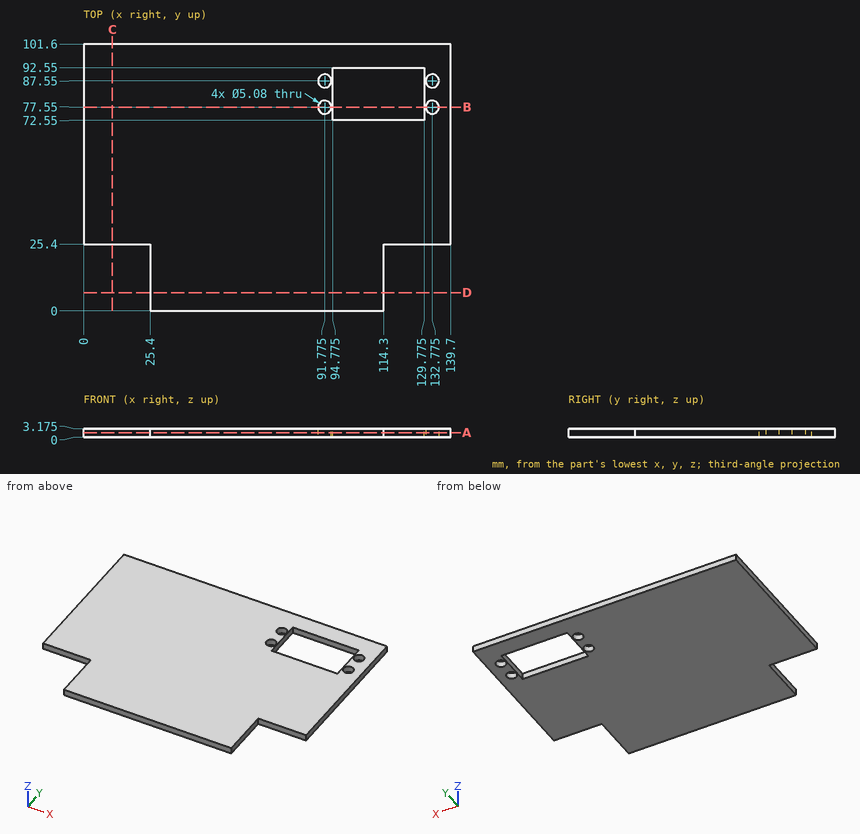
Job drawing, mm, ordinate dimensions from the low corner. One solid piece. Round coordinates to 2 decimals unless told otherwise and drop trailing zeros. Order: outer loops, then holes, each group sorted by start corner. A loop starts at its lowest first (then second) coordinate and runs counter-clockwise, first axis right, second up. Notation, with made-up numbers: M 88.25,28.5 L 129.25,28.5 A28 cw 129.25,59.5 Z; hole C -28,5.25 d10. An arc over 180 degrees is marked long. Write each question's results on one line, items separated by ' | '. Start each with the question number.
(1) Saw through at A-A, the plane z = 1.8. Give the cut face in (x, y) (3 decimals).
(2) Probe probe 1 along Y at (x, z) = (117, 2.3); probe 2 along Y at (x, z) = (94, 1.3); probe 3 along Y at (x, z) = (103.5, 0.4). List the from-to ranges inside material, lowest first. Write a range as from..to.
(3) Saw through at C-C, the plane x = 11. Give the cut face in (y, z) (3 decimals), then the cut area to 3 significant figures.
(4) Saw through at D-D, the plane y = 7. Give the cut face in (x, z) (3 decimals).
(5) Saw through at B-B, the plane y = 77.55. Give the cut face in (x, z) (3 decimals).
(6) Drop flat-ended pins along their axis: pin 1 (3 mm diameter, centred on x = 132.775, y = 77.55, fed in from -Z); pin 2 (1 mm diameter, centred on y = 77, z = 0.5, fed in from -X); pin 3 (1 mm diameter, centred on y = 10, z = 1, fed in from -X); pin 4 (1.6 mm diameter, centred on x = 130, z = 2, fed in from -Y). Give the stop position or say it passes through.
Established:
1) outline: M 0,25.4 L 25.4,25.4 L 25.4,0 L 114.3,0 L 114.3,25.4 L 139.7,25.4 L 139.7,101.6 L 0,101.6 Z; hole C 91.775,77.55 d5.08; hole C 91.775,87.55 d5.08; hole M 94.775,72.55 L 129.775,72.55 L 129.775,92.55 L 94.775,92.55 Z; hole C 132.775,77.55 d5.08; hole C 132.775,87.55 d5.08
2) probe 1: y = 25.4..72.55, 92.55..101.6 | probe 2: y = 0..76.32, 78.78..86.32, 88.78..101.6 | probe 3: y = 0..72.55, 92.55..101.6
3) outline: M 25.4,0 L 101.6,0 L 101.6,3.175 L 25.4,3.175 Z | area: 242 mm^2
4) outline: M 25.4,0 L 114.3,0 L 114.3,3.175 L 25.4,3.175 Z
5) outline: M 0,0 L 89.235,0 L 89.235,3.175 L 0,3.175 Z; M 94.315,0 L 94.775,0 L 94.775,3.175 L 94.315,3.175 Z; M 129.775,0 L 130.235,0 L 130.235,3.175 L 129.775,3.175 Z; M 135.315,0 L 139.7,0 L 139.7,3.175 L 135.315,3.175 Z
6) pin 1: passes through | pin 2: stops at x = 0 | pin 3: stops at x = 25.4 | pin 4: stops at y = 25.4
